Can you work these out from the drawing? Everything is in mm from the part's minimum corner. Round coordinates to 2 decimals unless told otherwise and drop trailing zeros. Write each loop counter-clockwise with the first axis right and the second up, starting at its lowest first coordinate (ties: lowest second). Pieces come first, ordered by that corner, then holes. Notation, with made-up numbers: M 24,51.25 L 77,51.25 A5 cw 77,57.25 Z; hole C 70,-12 d1. An arc over 180 degrees is marked long. Use one line per item in the form item = value. Start each with the question number.
Q1. I need wall thicknesses on line 1 along Y through (x, z) = (267, 13.75); line 2 along X through (y, z) = (380, 12); line 3 along Y through (x, z) = (862, 5). Which ranges of each line are inside material? Lowest first, please. Write a range as from..to.
Q2. I'm going to push a flat-ended pin straight in: pin 1 Ø12 at (y, z) = (724, 20) entering from +X. Where does the tip first touch, or does it pass through?
Q3. I want a section at B-B on z = 8.5. List the corners of the cut face in (x, y) for me.
Q4. I want a section at A-A on x = 234.5. List the corners of the cut face in (y, z) for me, and give its area (3 significant figures).
Q5. I want a section at C-C on y = 858. List the corners of the cut face in (x, z) for me.
Q6. I want a section at D-D on x = 981.5. List the corners of the cut face in (y, z) for me, and give its area (3 significant figures).
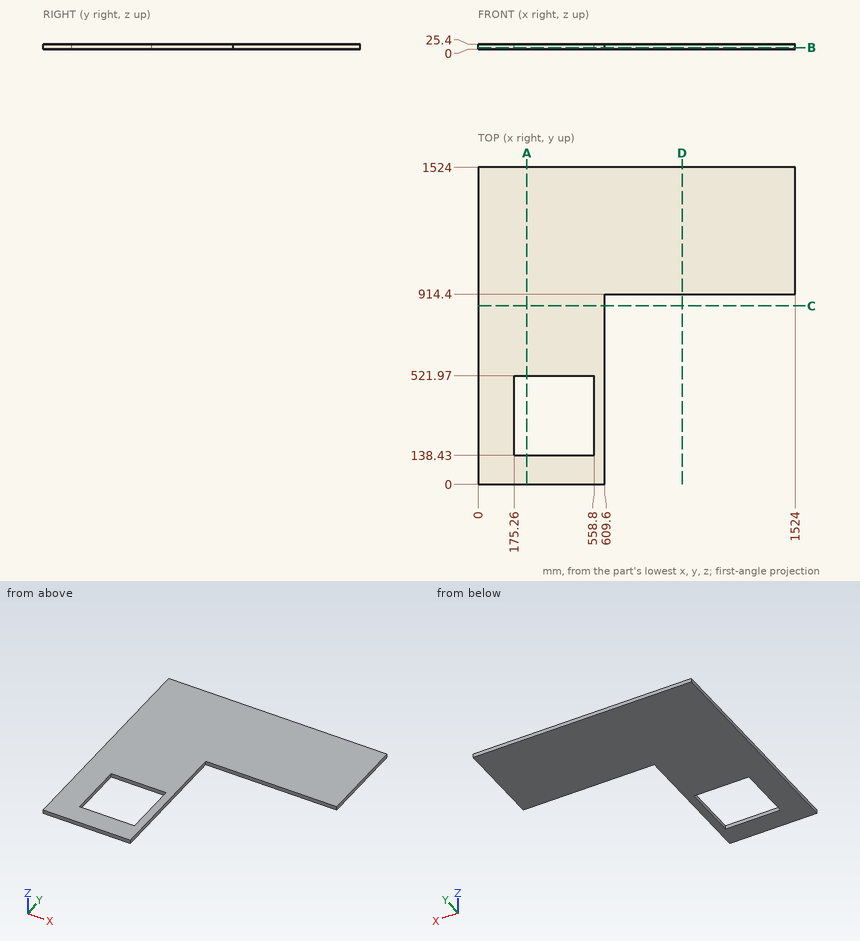
Reported:
q1.line_1 = 0..138.43, 521.97..1524
q1.line_2 = 0..175.26, 558.8..609.6
q1.line_3 = 914.4..1524
q2.pin_1 = 609.6
q3.outline = M 0,0 L 609.6,0 L 609.6,914.4 L 1524,914.4 L 1524,1524 L 0,1524 Z; hole M 175.26,138.43 L 558.8,138.43 L 558.8,521.97 L 175.26,521.97 Z
q4.outline = M 0,0 L 138.43,0 L 138.43,25.4 L 0,25.4 Z; M 521.97,0 L 1524,0 L 1524,25.4 L 521.97,25.4 Z
q4.area = 29,000 mm^2
q5.outline = M 0,0 L 609.6,0 L 609.6,25.4 L 0,25.4 Z
q6.outline = M 914.4,0 L 1524,0 L 1524,25.4 L 914.4,25.4 Z
q6.area = 15,500 mm^2
